The listing builds one solid part. Answer for the finished solid, in the listing's coordinates (mm). A direction names the side the tool comes from. Coordinates: 2 decimals unless noted, no trailing zeros. Order: outer loops, then holes, each group sorted by start corner. A loop starts at its lowest first (then second) coordinate and runs counter-clockwise, first axis right, second up. Notation, with made-up numbers: (2, -2) -> (47, -2) arc R21 cw to (47, 17) -> close; hole circle Ø3 at (50, 80.5). An arc over 180 degrees is marked (long way). Answer in a Markdown table with one row per item.
```python
from build123d import *

# Parameters (mm, degrees)
SKETCH1_W           = 130
SKETCH1_H           = 13
BOSS_EXTRUDE1_DEPTH = 37.17
SHELL1_T            = -2
SKETCH2_W           = 55
SKETCH2_H           = 2.13378228
CUT_EXTRUDE1_DEPTH  = 5
FILLET1_R           = 2


with BuildPart() as part:
    # Sketch1 → Boss-Extrude1 (new body)
    with BuildSketch(Plane.XY):
        with Locations((65, 6.5)):
            Rectangle(SKETCH1_W, SKETCH1_H)
    extrude(amount=-BOSS_EXTRUDE1_DEPTH)

    # Shell1
    shell1_openings = [part.faces().sort_by_distance(p)[0] for p in [
        (65, 0, -18.585),
    ]]
    offset(amount=SHELL1_T, openings=shell1_openings, kind=Kind.INTERSECTION)

    # Sketch2 → Cut-Extrude1 (cut)
    with BuildSketch(Plane.XY):
        with Locations((65, 1.06689114)):
            Rectangle(SKETCH2_W, SKETCH2_H)
    extrude(amount=-CUT_EXTRUDE1_DEPTH, mode=Mode.SUBTRACT)

    # Fillet1
    fillet1_edges = [part.edges().sort_by_distance(p)[0] for p in [
        (130, 6.5, -37.17),
        (0, 6.5, -37.17),
        (130, 6.5, 0),
        (0, 6.5, 0),
    ]]
    fillet(fillet1_edges, radius=FILLET1_R)


solid = part.part
```
(1) A cutting plane is placed at C-C, the plane x = 64. Determine the outline of the cut face in (y, z).
Check values:
| item | result |
|---|---|
| outline | (0, -37.17) -> (13, -37.17) -> (13, 0) -> (2.13, 0) -> (2.13, -2) -> (11, -2) -> (11, -35.17) -> (0, -35.17) -> close |
(2) A cutting plane is placed at B-B, the plane z = -12.5. Determine the outline of the cut face in (x, y), then the cut area to 3 significant figures.
Check values:
| item | result |
|---|---|
| outline | (0, 0) -> (2, 0) -> (2, 11) -> (128, 11) -> (128, 0) -> (130, 0) -> (130, 13) -> (0, 13) -> close |
| area | 304 mm² |
(3) Find the intervals of material crossed by line 1 along Z through (x, y) = (114, 9.25); line 2 along X through (y, z) = (7, -11); line 3 along Y through (x, z) = (110, -13), in increasing order. Write a range as from..to.
Check values:
| item | result |
|---|---|
| line 1 | -37.17..-35.17, -2..0 |
| line 2 | 0..2, 128..130 |
| line 3 | 11..13 |
(4) A cutting plane is placed at A-A, the plane y = 4.75. Determine the outline of the cut face in (x, z), then the cut area to 3 significant figures.
Check values:
| item | result |
|---|---|
| outline | (0, -35.17) arc R2 ccw to (2, -37.17) -> (128, -37.17) arc R2 ccw to (130, -35.17) -> (130, -2) arc R2 ccw to (128, 0) -> (2, 0) arc R2 ccw to (0, -2) -> close; hole (2, -35.17) -> (128, -35.17) -> (128, -2) -> (2, -2) -> close |
| area | 649 mm² |
(5) Which of the six approach directions +Z, -Z, +X, -X, +Y, -Y give full straight-line access (tool end or side, diameter ignored) to faces 1 (the flat face through (128, 5, -18)), 2 (the flat face through (0, 6, -18))?
Check values:
| item | result |
|---|---|
| face 1 | -Y |
| face 2 | +Z, -Z, -X, +Y, -Y |
(6) For a pull along X with two mould halves and no side action, classify faces 3 (the flat face through (130, 6, -18)), 4 (the flat face through (64, 11, -18)), 5 (the flat face through (64, 7, 0)), 6 (the flat face through (2, 5, -18)) as released by +X, released by -X, zero draft, split by the parting line, or undercut.
Check values:
| item | result |
|---|---|
| face 3 | released by +X |
| face 4 | undercut |
| face 5 | zero draft |
| face 6 | undercut |
(7) Flat-ended cylindrical pins translate along their axes: pin 1 (4 mm diameter, centred on x = 48.5, z = -29.5, fed in from -Y); pin 2 (2 mm diameter, centred on y = 1, z = -1, fed in from +X); pin 3 (2 mm diameter, centred on x = 52, z = -1.5, fed in from -Y). Find the tip coordinate at first contact, or state that the pin passes through.
Check values:
| item | result |
|---|---|
| pin 1 | y = 11 |
| pin 2 | x = 130 |
| pin 3 | y = 2.13 |
